Drawing for the job (mm, zero at the part's lowest x, y, z). Give positions to 0.01 mm unless a question says otherwise; leave off trailing zeros. Write each loop counter-clockwise with the first axis right and the second up, starting at its lowest first coordinate (ties: lowest second). Pieces come first, ordered by that corner, then holes. Notation, with made-up numbers: M 85.5,73.5 L 140.5,73.5 A23 cw 140.5,100.5 Z; hole C 27.25,41 d11. An arc over 180 degrees is marked long. Use CSV: the item, a comma, the result in double quotes. Start each with the question number.
1. Drill centre lines: line 1 along Y through (x, z) = (54.5, 2.5); line 2 along X through (y, z) = (50.5, 0.2); line 3 along Z through (x, y) = (24, 24). Where is each one in solid material? Low to high. Write a range as from..to.
2. Band-saw the part on A-A, the plane x = 31.25. List the corners of the cut face in (y, z), then the cut area to 3 significant figures.
3. Band-saw the part on C-C, the plane y = 5. List the corners of the cut face in (x, z), then the cut area to 3 significant figures.
4. Band-saw the part on B-B, the plane x = 9.5. List the corners of the cut face in (y, z).
5. Band-saw the part on D-D, the plane y = 36.5. List the corners of the cut face in (x, z), then the cut area to 3 significant figures.
6. Mould opens along Y. For the marked faces 1 and 2 say: pulls with the +Y half, pulls with the -Y half, needs draft (parallel to the pull), parting line crosses it, or undercut.
7. Drop a flat-ended pin along its axis: pin 1 Ø8 at (x, y) = (23, 39.5) entering from +Z. Give the stop position or say it passes through.
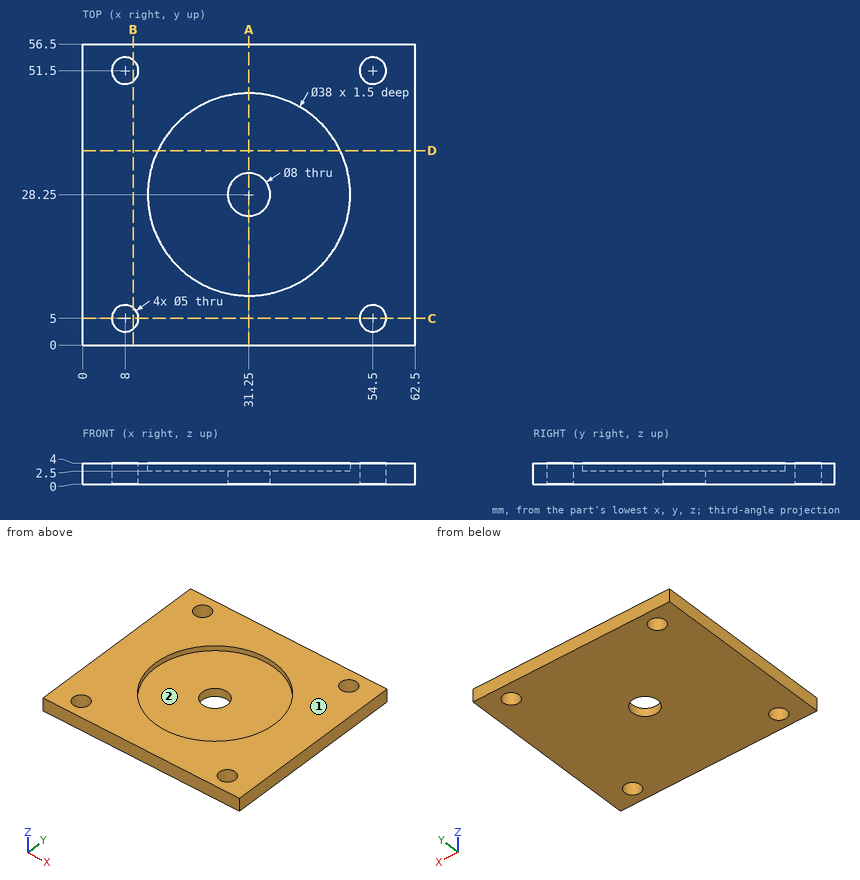
Output:
1,line 1,"y = 0..2.5, 7.5..49, 54..56.5"
1,line 2,"x = 0..5.71, 10.29..52.21, 56.79..62.5"
1,line 3,"z = 0..2.5"
2,outline,"M 0,0 L 24.25,0 L 24.25,2.5 L 9.25,2.5 L 9.25,4 L 0,4 Z; M 32.25,0 L 56.5,0 L 56.5,4 L 47.25,4 L 47.25,2.5 L 32.25,2.5 Z"
2,area,"149 mm²"
3,outline,"M 0,0 L 5.5,0 L 5.5,4 L 0,4 Z; M 10.5,0 L 52,0 L 52,4 L 10.5,4 Z; M 57,0 L 62.5,0 L 62.5,4 L 57,4 Z"
3,area,"210 mm²"
4,outline,"M 0,0 L 3,0 L 3,4 L 0,4 Z; M 7,0 L 49.5,0 L 49.5,4 L 7,4 Z; M 53.5,0 L 56.5,0 L 56.5,4 L 53.5,4 Z"
5,outline,"M 0,0 L 62.5,0 L 62.5,4 L 48.37,4 L 48.37,2.5 L 14.13,2.5 L 14.13,4 L 0,4 Z"
5,area,"199 mm²"
6,face 1,"needs draft"
6,face 2,"undercut"
7,pin 1,"stops at z = 2.5"
